Geometry check sheet. Reference: drawing and pictorial views, mm from the part's lowest x, y, z. A direction names the side the tool comes from. Round coordinates to 2 decimals unless told otherwise and drop trailing zeros. Order: outer loops, then holes, each group sorted by start corner. A loop starts at its lowest first (then second) coordinate and runs counter-clockwise, first axis right, second up.
(1) Release check for a two-part mould opening along X. For the marked faces 1, 2, 3 and 4 record: +X half, -X half, draft (parallel to the pull), parting line (faces both ways), or undercut.
(2) Sectioned sample at A-A (y = 21). Record the boundary of the cut face in (x, z).
(3) Material ranges on line 1 along Y through (x, z) = (55, 61.5) (1 decimal); line 2 along Z through (x, y) = (24.5, 13); line 3 along Z through (x, y) = (41, 23), recorded low to high.
(4) Set-up check for the marked faces 5, 6 and 7: record each of +Z, -Z, +X, -X, +Y, -Y from which the full face is reachable in a straight line by a thin tool's end or side.
(5) Sectioned sample at C-C (x = 29.5). Record the boundary of the cut face in (y, z) (1 decimal), plus the area to 3 significant figures.
(6) Go/stop test with flat-tipped pins: pin 1 (14.5 mm diameter, centred on x = 48.5, z = 49, fed in from +Y) (1 decimal); pin 2 (3 mm diameter, centred on x = 19.5, z = 44.5, fed in from -Y); pin 3 (4 mm diameter, centred on y = 15, z = 52.5, fed in from +X). Record where each tip stops, or that it passes through.
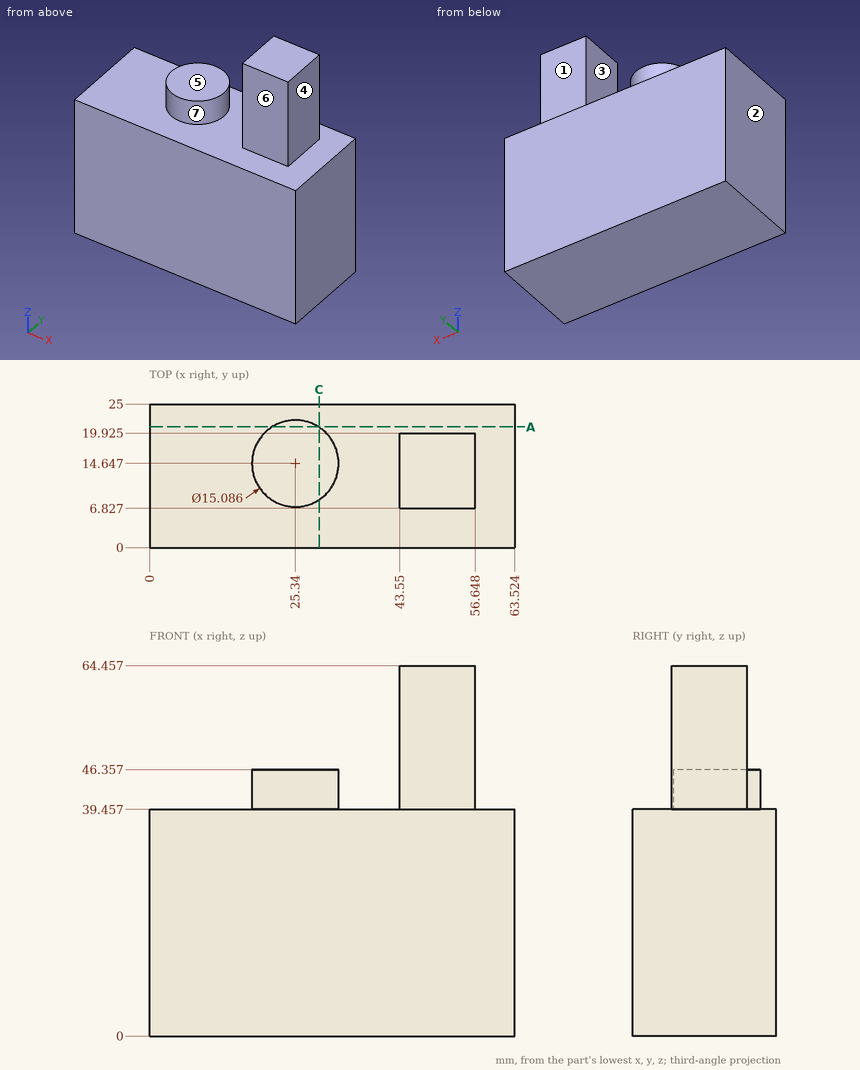
Answer below:
1. face 1: draft
1. face 2: -X half
1. face 3: undercut
1. face 4: +X half
2. outline: (0, 0) - (63.52, 0) - (63.52, 39.46) - (29.41, 39.46) - (29.41, 46.36) - (21.27, 46.36) - (21.27, 39.46) - (0, 39.46) - close
3. line 1: y = 6.8 to 19.9
3. line 2: z = 0 to 46.36
3. line 3: z = 0 to 39.46
4. face 5: +Z, -X, +Y, -Y
4. face 6: +Z, +X, -X, -Y
4. face 7: +Z
5. outline: (0, 0) - (25, 0) - (25, 39.5) - (20.9, 39.5) - (20.9, 46.4) - (8.4, 46.4) - (8.4, 39.5) - (0, 39.5) - close
5. area: 1,070 mm2
6. pin 1: stops at y = 19.9
6. pin 2: stops at y = 8.48
6. pin 3: stops at x = 56.65
